Read the model definition and answer for the solid it produces. Units are mm, in the model's axes. Give positions to 0.01 mm unless a question says otherwise; leave off trailing zeros. Loops run counter-clockwise (first coordinate to the right, second up) from the corner with the lowest first, then second, coordinate; pieces in that order, holes last. Notation, with made-up numbers: (28.25, 14) -> (70.25, 14) arc R17 ccw to (70.25, 26) -> close; hole circle Ø2 at (47, 68.5). An arc over 180 degrees is marked (long way). Answer as CSV lines item,"result". Start each with the question number.
```python
from build123d import *

# Parameters (mm, degrees)
SKETCH1_W           = 3
SKETCH1_H           = 3
SKETCH1_W_2         = 10
SKETCH1_H_2         = 5
BOSS_EXTRUDE4_DEPTH = 3


with BuildPart() as part:
    # Sketch1 → Boss-Extrude4 (new body)
    with BuildSketch(Plane.XY):
        Polygon((90, 201.25), (0, 0), (85, 0), (85, 7.26), (95, 7.26), (95, 0), (180, 0), align=None)
        with Locations((53.99, 61.857444444)):
            Rectangle(SKETCH1_W, SKETCH1_H, mode=Mode.SUBTRACT)
        with Locations((53.99, 71.157444444)):
            Rectangle(SKETCH1_W, SKETCH1_H, mode=Mode.SUBTRACT)
        with Locations((90, 89.737444444)):
            Rectangle(SKETCH1_W_2, SKETCH1_H_2, mode=Mode.SUBTRACT)
        with Locations((126.01, 62.967444444)):
            Rectangle(SKETCH1_W, SKETCH1_H, mode=Mode.SUBTRACT)
        with Locations((126.01, 72.267444444)):
            Rectangle(SKETCH1_W, SKETCH1_H, mode=Mode.SUBTRACT)
    extrude(amount=BOSS_EXTRUDE4_DEPTH)


solid = part.part
```
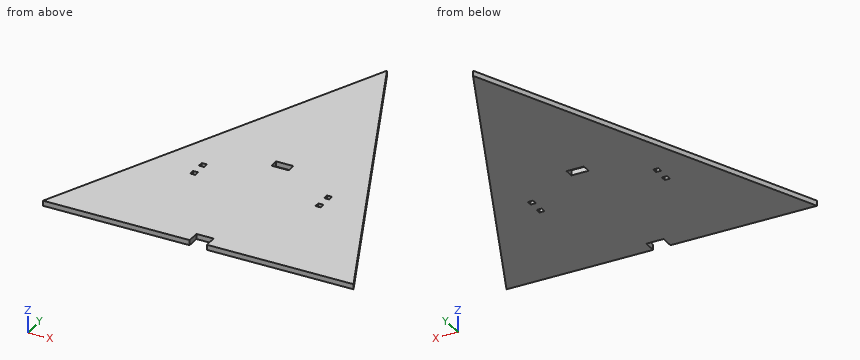
(1) Find the intervals of material crossed by line 1 along X through (y, z) = (63.5, 2.45); line 2 along X through (y, z) = (153, 0.95); line 3 along Y through (x, z) = (115.5, 0.9), in increasing order. Write a range as from..to.
(2) Find section B-B on x = 36. Write down the section's boundary in (y, z).
(3) Find section A-A on z = 0.9. Write down the section's boundary in (x, y), then the cut area to 3 significant figures.
(4) Find section C-C on y = 175.5. Write down the section's boundary in (x, z).
(5) Each of these flat-tipped pins is pushed along its axis until it touches: P1, Ø1.5, axis at y = 89.5, z = 1, coming from the -X side; P2, Ø0.9, axis at x = 126, z = 1.5, coming from the +Y side; P3, Ø0.9, axis at y = 71.5, z = 2, coming from the -X side. Where does it stop, or does it pass through?
Answer block:
1,line 1,"x = 28.4..124.51, 127.51..151.6"
1,line 2,"x = 68.42..111.58"
1,line 3,"y = 0..144.23"
2,outline,"(0, 0) -> (80.5, 0) -> (80.5, 3) -> (0, 3) -> close"
3,outline,"(0, 0) -> (85, 0) -> (85, 7.26) -> (95, 7.26) -> (95, 0) -> (180, 0) -> (90, 201.25) -> close; hole (52.49, 60.36) -> (55.49, 60.36) -> (55.49, 63.36) -> (52.49, 63.36) -> close; hole (52.49, 69.66) -> (55.49, 69.66) -> (55.49, 72.66) -> (52.49, 72.66) -> close; hole (85, 87.24) -> (95, 87.24) -> (95, 92.24) -> (85, 92.24) -> close; hole (124.51, 61.47) -> (127.51, 61.47) -> (127.51, 64.47) -> (124.51, 64.47) -> close; hole (124.51, 70.77) -> (127.51, 70.77) -> (127.51, 73.77) -> (124.51, 73.77) -> close"
3,area,"18,000 mm2"
4,outline,"(78.48, 0) -> (101.52, 0) -> (101.52, 3) -> (78.48, 3) -> close"
5,P1,"stops at x = 39.69"
5,P2,"stops at y = 121.76"
5,P3,"stops at x = 31.77"
